Design review of the part built by this model. Coordinates are the model's own, in mm. A direction names the side the tool comes from. Coordinates: 2 decimals unless noted, no trailing zeros. Loops run counter-clockwise (first coordinate to the right, second up) from the corner with the lowest first, then second, coordinate; pieces in that order, holes last.
Q1. Add section C-C on x = 3.75. Give the boundary of the cut face in (y, z).
Q2. Draft analysis for pull direction X (two halves, no side actions). For faces 4 (the face through (0.16, -0.9, 0.86)), 5 (the face through (10.93, -0.76, 24.4)), 6 (the face through (0, -1, 20)), 7 (the face through (0, -1, 17)), state which applies: released by +X, released by -X, zero draft, split by the parting line, or undercut.
Q3. Wall thickness on probe 1 along Y at (x, z) = (0, 0.4); probe 2 along Z at (x, y) = (-5.25, -13.5); probe 3 along Y at (x, z) = (1, 7.25): over which ranges is each line inside the solid? List them lowest first.
Q4. Add section A-A on y = -11.5. Give the boundary of the cut face in (x, z).
Q5. Machinability: for faces 1 (the face through (-6.5, -0.8, 18.5)), 2 (the face through (0, -1.5, 14)), 3 (the face through (0, -20, 1)), which of the approach directions +Z, -Z, +X, -X, +Y, -Y give a long, thin tool a straight path to every point of the face, cutting with its end or side? Answer none if there is none.
Q6. For P1, Ø3, axis at x = -1.5, y = -17.5, coming from the +Z side; P2, Ø4.5, axis at x = 0, y = -11.5, coming from the +Z side, all flat-tipped, find the tip position at first contact; note any pin that passes through.
Q7. Add section B-B on z = 18.5. Give the boundary of the cut face in (x, y), and give its area (3 significant figures).
Q8. Add section D-D on x = -1.5. Give the boundary of the cut face in (y, z), and give its area (3 significant figures).
```python
from build123d import *

# Parameters (mm, degrees)
F1_DEPTH = 11.5
F2_R     = 2.5
F3_DEPTH = 25
F5_DEPTH = 25
F6_R     = 2


with BuildPart() as f1:
    # F0 (on Right) → F1 (new body, symmetric)
    with BuildSketch(Plane.YZ):
        with BuildLine():
            ThreePointArc((-3, 0), (-0.87868, 0.87868), (0, 3))
            Line((0, 3), (0, 25))
            Line((0, 25), (-1.5, 25))
            Line((-1.5, 25), (-1.5, 3))
            ThreePointArc((-1.5, 3), (-1.93934, 1.93934), (-3, 1.5))
            Line((-3, 1.5), (-20, 1.5))
            Line((-20, 1.5), (-20, 0))
            Line((-20, 0), (-3, 0))
        make_face()
    extrude(amount=F1_DEPTH, both=True)

    # F2 (on face) → F3 (cut)
    with BuildSketch(Plane.XY.offset(1.5)):
        with Locations((0, -11.5)):
            Circle(F2_R)
    extrude(amount=-F3_DEPTH, mode=Mode.SUBTRACT)

    # F4 (on face) → F5 (cut)
    with BuildSketch(Plane.XZ.offset(1.5)):
        with BuildLine():
            Line((5, 20), (-5, 20))
            ThreePointArc((-5, 20), (-6.5, 18.5), (-5, 17))
            Line((-5, 17), (5, 17))
            ThreePointArc((5, 17), (6.5, 18.5), (5, 20))
        make_face()
    extrude(amount=-F5_DEPTH, mode=Mode.SUBTRACT)

    # F6
    f6_edges = [f1.edges().sort_by_distance(p)[0] for p in [
        (11.5, -0.75, 25),
        (-11.5, -0.75, 25),
        (11.5, -20, 0.75),
        (-11.5, -20, 0.75),
    ]]
    fillet(f6_edges, radius=F6_R)


solid = f1.part
```
Entries:
1. outline: (-20, 0) - (-3, 0) arc R3 ccw to (0, 3) - (0, 17) - (-1.5, 17) - (-1.5, 3) arc R1.5 cw to (-3, 1.5) - (-20, 1.5) - close; (-1.5, 20) - (0, 20) - (0, 25) - (-1.5, 25) - close
2. face 4: zero draft
2. face 5: released by +X
2. face 6: undercut
2. face 7: undercut
3. probe 1: y = -20 to -14, -9 to -1.5
3. probe 2: z = 0 to 1.5
3. probe 3: y = -1.5 to 0
4. outline: (-11.5, 0) - (-2.5, 0) - (-2.5, 1.5) - (-11.5, 1.5) - close; (2.5, 0) - (11.5, 0) - (11.5, 1.5) - (2.5, 1.5) - close
5. face 1: +Y, -Y
5. face 2: +Z, +X, -X, -Y
5. face 3: +Z, -Z, +X, -X, -Y
6. P1: stops at z = 1.5
6. P2: passes through
7. outline: (-11.5, -1.5) - (-6.5, -1.5) - (-6.5, 0) - (-11.5, 0) - close; (6.5, -1.5) - (11.5, -1.5) - (11.5, 0) - (6.5, 0) - close
7. area: 15.0 mm2
8. outline: (-20, 0) - (-13.5, 0) - (-13.5, 1.5) - (-20, 1.5) - close; (-9.5, 0) - (-3, 0) arc R3 ccw to (0, 3) - (0, 17) - (-1.5, 17) - (-1.5, 3) arc R1.5 cw to (-3, 1.5) - (-9.5, 1.5) - close; (-1.5, 20) - (0, 20) - (0, 25) - (-1.5, 25) - close
8. area: 53.3 mm2
